The model under review builds one solid part; all positions refer to its coordinate system, in mm. A direction names the side the tool comes from. Give positions to 0.01 mm unless a question says otherwise; leave off trailing zeros. Order: outer loops, then holes, each group sorted by start corner. A loop starts at its lowest first (then second) coordinate and runs counter-clockwise, first axis right, second up. Notation, with made-up numbers: (76.5, 30) - (98.5, 30) arc R19 cw to (98.5, 52) - close; hole circle Ø3 at (-32.5, 63.25). An arc over 180 degrees is marked (long way). Write item = value, one per line. Start each with the question number.
1. We need section C-C, the plane x = 73. Give the boundary of the cut face in (y, z).
2. For P1, Ø10, axis at y = 19, z = -10.5, coming from the +X side; P2, Ø2.5, axis at x = 50, z = -44.5, coming from the +Y side; P3, Ø4, axis at x = 49, z = -56, coming from the +Y side; P4, Ø1.5, axis at x = 24.5, z = -43, coming from the +Y side, all flat-tipped, find the tip position at first contact; note any pin that passes through.
3. We need section D-D, the plane x = 50. State how many separate pieces and enclosed holes the cut face has, and give its area (4 significant figures).
4. We need section A-A, the plane z = -55.5. Give the boundary of the cut face in (x, y), and give its area (3 significant figures).
5. Wall thickness on probe 1 along Z at (x, y) = (49, 33.5); probe 2 along Y at (x, z) = (10, -53); probe 3 along X at (y, z) = (7, -44.5): over which ranges is each line inside the solid? List them lowest first.
6. Mouldability with a two-part tool opening along X and no side actions: class faces 1 (the flat face through (50, 32, -37.5)), 2 (the cylindrical face through (49.04, 22.68, -42.19)), 3 (the cylindrical face through (14, 15.07, -86.07)), 4 (the flat face through (49, 10, -54)) as pulls with the +X half, pulls with the -X half, needs draft (parallel to the pull), parting line crosses it, or undercut.
7. We need section B-B, the plane y = 16.5. Give the boundary of the cut face in (x, z).
8. Machinability: for faces 5 (the flat face through (94, 10, -51)), 6 (the cylindrical face through (38.93, 32.53, -61)), 7 (the cylindrical face through (61, 32.53, -61.07)), which of the approach directions +Z, -Z, +X, -X, +Y, -Y give a long, thin tool a straight path to every point of the face, cutting with its end or side? Answer none if there is none.
from build123d import *

# Parameters (mm, degrees)
SKETCH1_W           = 100
SKETCH1_H           = 100
BOSS_EXTRUDE1_DEPTH = 10
SKETCH2_W           = 75
SKETCH2_H           = 75
BOSS_EXTRUDE2_DEPTH = 10
SKETCH3_W           = 50
SKETCH3_H           = 50
BOSS_EXTRUDE3_DEPTH = 10
SKETCH4_W           = 25
SKETCH4_H           = 25
BOSS_EXTRUDE4_DEPTH = 5
SKETCH5_R           = 2.5
CUT_EXTRUDE1_DEPTH  = 25
SKETCH6_R           = 1.5
CUT_EXTRUDE2_DEPTH  = 10
FILLET2_R           = 5


with BuildPart() as part:
    # Sketch1 → Boss-Extrude1 (new body)
    with BuildSketch(Plane(origin=(0, 0, 0), x_dir=(1, 0, 0), z_dir=(0, 1, 0))):
        with Locations((50, 50)):
            Rectangle(SKETCH1_W, SKETCH1_H)
    extrude(amount=BOSS_EXTRUDE1_DEPTH)

    # Sketch2 → Boss-Extrude2 (add)
    with BuildSketch(Plane(origin=(0, 10, 0), x_dir=(1, 0, 0), z_dir=(0, 1, 0))):
        with Locations((50, 50)):
            Rectangle(SKETCH2_W, SKETCH2_H)
    extrude(amount=BOSS_EXTRUDE2_DEPTH)

    # Sketch3 → Boss-Extrude3 (add)
    with BuildSketch(Plane(origin=(0, 20, 0), x_dir=(1, 0, 0), z_dir=(0, 1, 0))):
        with Locations((50, 50)):
            Rectangle(SKETCH3_W, SKETCH3_H)
    extrude(amount=BOSS_EXTRUDE3_DEPTH)

    # Sketch4 → Boss-Extrude4 (add)
    with BuildSketch(Plane(origin=(0, 30, 0), x_dir=(1, 0, 0), z_dir=(0, 1, 0))):
        with Locations((50, 50)):
            Rectangle(SKETCH4_W, SKETCH4_H)
    extrude(amount=BOSS_EXTRUDE4_DEPTH)

    # Sketch5 → Cut-Extrude1 (cut)
    with BuildSketch(Plane(origin=(0, 35, 0), x_dir=(1, 0, 0), z_dir=(0, 1, 0))):
        with Locations(Location((50, 55.5, 0), (0, 0, 270))):
            Circle(SKETCH5_R)
        with Locations(Location((50, 44.5, 0), (0, 0, 270))):
            Circle(SKETCH5_R)
    extrude(amount=-CUT_EXTRUDE1_DEPTH, mode=Mode.SUBTRACT)

    # Sketch6 → Cut-Extrude2 (cut)
    with BuildSketch(Plane(origin=(0, 10, 0), x_dir=(1, 0, 0), z_dir=(0, 1, 0))):
        with Locations(Location((50, 55.5, 0), (0, 0, 270))):
            Circle(SKETCH6_R)
        with Locations(Location((50, 44.5, 0), (0, 0, 270))):
            Circle(SKETCH6_R)
    extrude(amount=-CUT_EXTRUDE2_DEPTH, mode=Mode.SUBTRACT)

    # Fillet2
    fillet2_edges = [part.edges().sort_by_distance(p)[0] for p in [
        (12.5, 15, -87.5),
        (12.5, 15, -12.5),
        (87.5, 15, -12.5),
        (87.5, 15, -87.5),
        (37.5, 32.5, -62.5),
        (37.5, 32.5, -37.5),
        (62.5, 32.5, -37.5),
        (62.5, 32.5, -62.5),
    ]]
    fillet(fillet2_edges, radius=FILLET2_R)


solid = part.part
Model answer:
q1.outline = (0, -100) - (10, -100) - (10, -87.5) - (20, -87.5) - (20, -75) - (30, -75) - (30, -25) - (20, -25) - (20, -12.5) - (10, -12.5) - (10, 0) - (0, 0) - close
q2.P1 = 87.08
q2.P2 = through
q2.P3 = 35
q2.P4 = 30
q3.separate_pieces = 3
q3.enclosed_holes = 0
q3.area = 2,065 mm2
q4.outline = (0, 0) - (48.5, 0) - (48.5, 10) - (47.5, 10) - (47.5, 35) - (37.5, 35) - (37.5, 30) - (25, 30) - (25, 20) - (12.5, 20) - (12.5, 10) - (0, 10) - close; (51.5, 0) - (100, 0) - (100, 10) - (87.5, 10) - (87.5, 20) - (75, 20) - (75, 30) - (62.5, 30) - (62.5, 35) - (52.5, 35) - (52.5, 10) - (51.5, 10) - close
q4.area = 2,220 mm2
q5.probe_1 = -62.5 to -57.79, -53.21 to -46.79, -42.21 to -37.5
q5.probe_2 = 0 to 10
q5.probe_3 = 0 to 48.5, 51.5 to 100
q6.face_1 = needs draft
q6.face_2 = undercut
q6.face_3 = pulls with the -X half
q6.face_4 = undercut
q7.outline = (12.5, -82.5) arc R5 ccw to (17.5, -87.5) - (82.5, -87.5) arc R5 ccw to (87.5, -82.5) - (87.5, -17.5) arc R5 ccw to (82.5, -12.5) - (17.5, -12.5) arc R5 ccw to (12.5, -17.5) - close; hole circle Ø5 at (50, -55.5); hole circle Ø5 at (50, -44.5)
q8.face_5 = +Y
q8.face_6 = -Z, -X, +Y
q8.face_7 = -Z, +X, +Y
